Design review of the part built by this model. Coordinates are the model's own, in mm. Give positions to 0.01 mm unless a question says otherwise; leave off trailing zeros. Write each loop counter-clockwise with the first axis right and the second up, starting at its lowest first coordinate (ties: lowest second). Pieces come first, ordered by that corner, then holes. Notation, with made-up numbers: M 1.25,7 L 36.25,7 A31 cw 36.25,43 Z; hole C 36.5,1 d1. An arc over 180 degrees is marked long. Use a Markdown table: item, result. Add a question column.
```python
from build123d import *

# Parameters (mm, degrees)
SKETCH1_W                       = 274.5232
SKETCH1_H                       = 171.45
BOSS_EXTRUDE1_DEPTH             = 9.525
F_9_32_0_28125_DIAMETER_HOLE1_D = 7.14375
CHAMFER1_SIZE                   = 0.762
CUT_EXTRUDE1_DEPTH              = 10.525


with BuildPart() as part:
    # Sketch1 → Boss-Extrude1 (new body)
    with BuildSketch(Plane.XY):
        with Locations((137.2616, 85.725)):
            Rectangle(SKETCH1_W, SKETCH1_H)
    extrude(amount=BOSS_EXTRUDE1_DEPTH)

    # 9/32 (0.28125) Diameter Hole1 (through all)
    with Locations(Plane.XY.offset(9.525)):
        with Locations((6.0198, 84.1248), (12.3698, 133.35), (12.3698, 31.75), (267.5382, 133.35), (267.5382, 84.1248), (267.5382, 31.75)):
            Hole(F_9_32_0_28125_DIAMETER_HOLE1_D / 2)

    # Chamfer1
    chamfer1_edges = [part.edges().sort_by_distance(p)[0] for p in [
        (137.2616, 171.45, 9.525),
        (137.2616, 171.45, 0),
        (137.2616, 0, 0),
        (137.2616, 0, 9.525),
    ]]
    chamfer(chamfer1_edges, length=CHAMFER1_SIZE)

    # Sketch6 → Cut-Extrude1 (cut, through all)
    with BuildSketch(Plane.XY.offset(9.525)):
        with BuildLine():
            Line((33.381181438, 139.082261479), (110.606344338, 93.948517799))
            ThreePointArc((110.606344338, 93.948517799), (115.325162901, 85.725), (110.606344338, 77.501482201))
            Line((110.606344338, 77.501482201), (33.381181438, 32.367738521))
            ThreePointArc((33.381181438, 32.367738521), (23.834391031, 32.329764227), (19.05, 40.591256319))
            Line((19.05, 40.591256319), (19.05, 130.858743681))
            ThreePointArc((19.05, 130.858743681), (23.834391031, 139.120235773), (33.381181438, 139.082261479))
        make_face()
        with BuildLine():
            Line((62.002810809, 137.064482201), (132.455418562, 95.888914284))
            ThreePointArc((132.455418562, 95.888914284), (137.2616, 94.587432082), (142.067781438, 95.888914284))
            Line((142.067781438, 95.888914284), (212.520389191, 137.064482201))
            ThreePointArc((212.520389191, 137.064482201), (216.908081584, 147.777640332), (207.714207753, 154.813))
            Line((207.714207753, 154.813), (66.808992247, 154.813))
            ThreePointArc((66.808992247, 154.813), (57.615118416, 147.777640332), (62.002810809, 137.064482201))
        make_face()
        with BuildLine():
            Line((241.142018562, 139.082261479), (163.916855662, 93.948517799))
            ThreePointArc((163.916855662, 93.948517799), (159.198037099, 85.725), (163.916855662, 77.501482201))
            Line((163.916855662, 77.501482201), (241.142018562, 32.367738521))
            ThreePointArc((241.142018562, 32.367738521), (250.688808969, 32.329764227), (255.4732, 40.591256319))
            Line((255.4732, 40.591256319), (255.4732, 130.858743681))
            ThreePointArc((255.4732, 130.858743681), (250.688808969, 139.120235773), (241.142018562, 139.082261479))
        make_face()
        with BuildLine():
            Line((66.808992247, 16.637), (207.714207753, 16.637))
            ThreePointArc((207.714207753, 16.637), (216.908081584, 23.672359668), (212.520389191, 34.385517799))
            Line((212.520389191, 34.385517799), (142.067781438, 75.561085716))
            ThreePointArc((142.067781438, 75.561085716), (137.2616, 76.862567918), (132.455418562, 75.561085716))
            Line((132.455418562, 75.561085716), (62.002810809, 34.385517799))
            ThreePointArc((62.002810809, 34.385517799), (57.615118416, 23.672359668), (66.808992247, 16.637))
        make_face()
    extrude(amount=-CUT_EXTRUDE1_DEPTH, mode=Mode.SUBTRACT)


solid = part.part
```
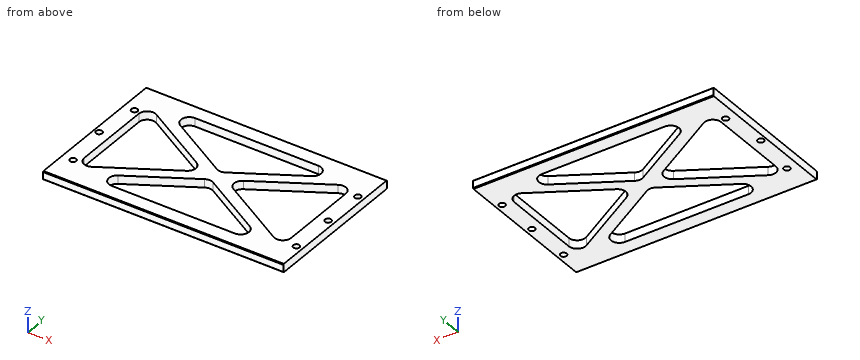
(1) Add section C-C on y = 125. Give the number of separate pieces and of enclosed holes in the cut face, then the cut area to 3 significant figures.
(2) Add section D-D on x = 85.5. Give the boundary of the cut face in (y, z) (3 decimals).
(3) Add section B-B on x = 127. Give the boundary of the cut face in (y, z) (3 decimals), then the cut area to 3 significant figures.
(4) Add section A-A on y = 91. Give the boundary of the cut face in (x, z) (3 decimals).
(5) Wall thickness on L1, parallel to Y at x = 110.5, z = 9; L2, parallel to Y at x = 173, z = 1.5; L3, parallel to X at y = 81, z = 8.75: over which ranges is each line inside the solid? List them lowest first.
From the geometry:
| question | item | result |
|---|---|---|
| 1 | separate pieces | 4 |
| 1 | enclosed holes | 0 |
| 1 | area | 842 mm^2 |
| 2 | outline | M 0,0.762 L 0.762,0 L 16.637,0 L 16.637,9.525 L 0.762,9.525 L 0,8.763 Z; M 48.118,0 L 62.828,0 L 62.828,9.525 L 48.118,9.525 Z; M 108.622,0 L 123.332,0 L 123.332,9.525 L 108.622,9.525 Z; M 154.813,0 L 170.688,0 L 171.45,0.762 L 171.45,8.763 L 170.688,9.525 L 154.813,9.525 Z |
| 3 | outline | M 0,0.762 L 0.762,0 L 16.637,0 L 16.637,9.525 L 0.762,9.525 L 0,8.763 Z; M 72.373,0 L 99.077,0 L 99.077,9.525 L 72.373,9.525 Z; M 154.813,0 L 170.688,0 L 171.45,0.762 L 171.45,8.763 L 170.688,9.525 L 154.813,9.525 Z |
| 3 | area | 570 mm^2 |
| 4 | outline | M 0,0 L 19.05,0 L 19.05,9.525 L 0,9.525 Z; M 113.731,0 L 160.792,0 L 160.792,9.525 L 113.731,9.525 Z; M 255.473,0 L 274.523,0 L 274.523,9.525 L 255.473,9.525 Z |
| 5 | L1 | y = 0.24 to 16.64, 62.73 to 77.44, 94.01 to 108.72, 154.81 to 171.21 |
| 5 | L2 | y = 0 to 16.64, 57.48 to 72.19, 99.26 to 113.97, 154.81 to 171.45 |
| 5 | L3 | x = 0 to 4.29, 7.75 to 19.05, 114.07 to 160.45, 255.47 to 265.81, 269.27 to 274.52 |
